```python
from build123d import *

# Parameters (mm, degrees)
BOSS_EXTRUDE1_DEPTH = 4.5
SKETCH3_W           = 3
SKETCH3_H           = 1
SKETCH3_W_2         = 1
SKETCH3_H_2         = 2
EXTRUDE_THIN1_DEPTH = 5


with BuildPart() as part:
    # Sketch1 → Boss-Extrude1 (new body)
    with BuildSketch(Plane(origin=(0, 0, 0), x_dir=(1, 0, 0), z_dir=(0, 1, 0))):
        Polygon((0, 12), (0, 18), (26.7, 18), (26.7, 0), (0, 0), (0, 6), (22.7, 6), (22.7, 12), align=None)
    extrude(amount=BOSS_EXTRUDE1_DEPTH)

    # Sketch3 → Extrude-Thin1 (add)
    with BuildSketch(Plane.ZY):
        with Locations((-15, 2.25)):
            Rectangle(SKETCH3_W, SKETCH3_H)
        with Locations((-15, 2.25)):
            Rectangle(SKETCH3_W_2, SKETCH3_H_2)
        with Locations((-3, 2.25)):
            Rectangle(SKETCH3_W_2, SKETCH3_H_2)
        with Locations((-3, 2.25)):
            Rectangle(SKETCH3_W, SKETCH3_H)
    extrude(amount=EXTRUDE_THIN1_DEPTH)


solid = part.part
```
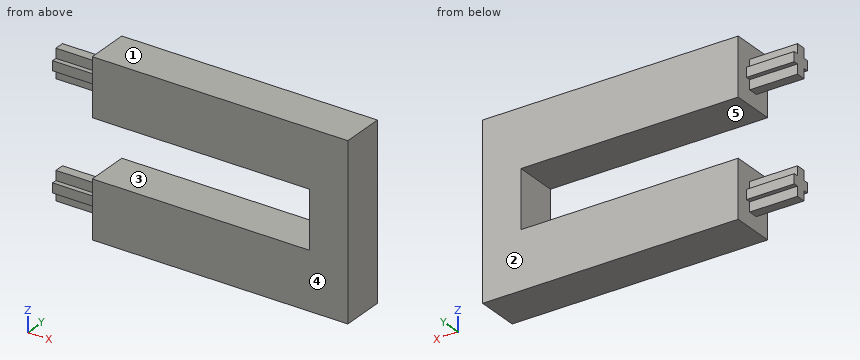
Can you work these out from the model? Positions are in its coordinate system, mm. Face numbers are marked on the shaded views. A direction names the side the tool comes from. Round coordinates to 2 decimals unless told otherwise and drop trailing zeros. Order: outer loops, then holes, each group sorted by start corner. A loop starts at its lowest first (then second) coordinate and runs counter-clockwise, first axis right, second up. Notation, with made-up numbers: (45, 37.25) -> (55, 37.25) arc R11 ccw to (55, 48.25) -> close; hole circle Ø7 at (-3, -35.5). An arc over 180 degrees is marked (long way). Return JSON: item names as keys, results as strings. Group by question number.
1. If we section it at A-A, the plane x = -3: Write out the boundary of the cut face in (y, z).
2. I need wall thicknesses on line 1 (Z direction, x = 20, y = 1.55); line 2 (X direction, y = 3.6, z = -12.5); line 3 (X direction, y = 3.35, z = -11.25). Which ranges of each line are inside material? Lowest first, please. Write a range as [from, to].
3. Will these pins go through, and if not, where does the flat tip stop? pin 1 (0.8 mm diameter, centred on x = -2.5, z = -2, fed in from -Y); pin 2 (0.6 mm diameter, centred on x = -2.5, y = 3, fed in from +Z); pin 3 (1.1 mm diameter, centred on x = -2, z = -4, fed in from -Y).
4. If we section it at C-C, the plane y = 4: Write out the boundary of the cut face in (x, z).
5. If we section it at D-D, the plane x = 12: Write out the boundary of the cut face in (y, z), then the cut area to 3 significant figures.
6. Which directions (+Z, -Z, +X, -X, +Y, -Y) give clear straight access to the entire face, cutting with the end or side of a thin tool? Please do the marked faces 4 and 5.
7. We'd pull the mould along Z, two halves only. Please class the marked faces 1, 2 and 3: released by +Z, released by -Z, zero draft, split by the parting line, or undercut.
8. If we section it at B-B, the plane z = -3: Write out the boundary of the cut face in (x, y), then the cut area to 3 significant figures.
Output values:
{
 "1": {"outline": "(1.25, -15.5) -> (1.75, -15.5) -> (1.75, -16.5) -> (2.75, -16.5) -> (2.75, -15.5) -> (3.25, -15.5) -> (3.25, -14.5) -> (2.75, -14.5) -> (2.75, -13.5) -> (1.75, -13.5) -> (1.75, -14.5) -> (1.25, -14.5) -> close; (1.25, -3.5) -> (1.75, -3.5) -> (1.75, -4.5) -> (2.75, -4.5) -> (2.75, -3.5) -> (3.25, -3.5) -> (3.25, -2.5) -> (2.75, -2.5) -> (2.75, -1.5) -> (1.75, -1.5) -> (1.75, -2.5) -> (1.25, -2.5) -> close"},
 "2": {"line 1": "[-18, -12], [-6, 0]", "line 2": "[0, 26.7]", "line 3": "[22.7, 26.7]"},
 "3": {"pin 1": "y = 1.75", "pin 2": "z = -1.5", "pin 3": "y = 1.25"},
 "4": {"outline": "(0, -18) -> (26.7, -18) -> (26.7, 0) -> (0, 0) -> (0, -6) -> (22.7, -6) -> (22.7, -12) -> (0, -12) -> close"},
 "5": {"outline": "(0, -18) -> (4.5, -18) -> (4.5, -12) -> (0, -12) -> close; (0, -6) -> (4.5, -6) -> (4.5, 0) -> (0, 0) -> close", "area": "54.0 mm²"},
 "6": {"face 4": "+Z, -Z, +X, -X, -Y", "face 5": "-X, +Y, -Y"},
 "7": {"face 1": "released by +Z", "face 2": "zero draft", "face 3": "undercut"},
 "8": {"outline": "(-5, 1.25) -> (0, 1.25) -> (0, 0) -> (26.7, 0) -> (26.7, 4.5) -> (0, 4.5) -> (0, 3.25) -> (-5, 3.25) -> close", "area": "130 mm²"}
}
